from build123d import *

# Parameters (mm, degrees)
SKETCH1_R           = 3.2
BOSS_EXTRUDE1_DEPTH = 20
SKETCH3_R           = 3.2
CUT_EXTRUDE1_DEPTH  = 10
CUT_EXTRUDE2_DEPTH  = 5.5
SKETCH6_R           = 1.5
CUT_EXTRUDE4_DEPTH  = 21
CHAMFER1_SIZE       = 2
SKETCH8_R           = 1.16
CUT_EXTRUDE5_DEPTH  = 10
FILLET1_R           = 1


with BuildPart() as part:
    # Sketch1 → Boss-Extrude1 (new body)
    with BuildSketch(Plane.XY):
        with BuildLine():
            Line((20.020647688, -81), (9.925461516, 1.218693434))
            ThreePointArc((9.925461516, 1.218693434), (0, 10), (-9.925461516, 1.218693434))
            Line((-9.925461516, 1.218693434), (-20.020647688, -81))
            Line((-20.020647688, -81), (-42.020647688, -81))
            Line((-42.020647688, -81), (-42.020647688, -90))
            Line((-42.020647688, -90), (42.020647688, -90))
            Line((42.020647688, -90), (42.020647688, -81))
            Line((42.020647688, -81), (20.020647688, -81))
        make_face()
        Circle(SKETCH1_R, mode=Mode.SUBTRACT)
    extrude(amount=BOSS_EXTRUDE1_DEPTH)

    # Sketch3 → Cut-Extrude1 (cut, through all)
    with BuildSketch(Plane(origin=(0, -81, 0), x_dir=(1, 0, 0), z_dir=(0, 1, 0))):
        with Locations((-31.020647688, -10)):
            Circle(SKETCH3_R)
        with Locations((31.020647688, -10)):
            Circle(SKETCH3_R)
    extrude(amount=-CUT_EXTRUDE1_DEPTH, mode=Mode.SUBTRACT)

    # Sketch4 → Cut-Extrude2 (cut)
    with BuildSketch(Plane.XY.offset(20)):
        Polygon((0, 6.062177826), (-5.25, 3.031088913), (-5.25, -3.031088913), (0, -6.062177826), (5.25, -3.031088913), (5.25, 3.031088913), align=None)
    extrude(amount=-CUT_EXTRUDE2_DEPTH, mode=Mode.SUBTRACT)

    # Sketch6 → Cut-Extrude4 (cut, through all)
    with BuildSketch(Plane.XY.offset(20)):
        with Locations((0, -66)):
            Circle(SKETCH6_R)
        with Locations((0, -74)):
            Circle(SKETCH6_R)
        with Locations((0, -82)):
            Circle(SKETCH6_R)
    extrude(amount=-CUT_EXTRUDE4_DEPTH, mode=Mode.SUBTRACT)

    # Chamfer1
    chamfer1_edges = [part.edges().sort_by_distance(p)[0] for p in [
        (-1.5, -66, 20),
        (-1.5, -74, 20),
        (-1.5, -82, 20),
    ]]
    chamfer(chamfer1_edges, length=CHAMFER1_SIZE)

    # Sketch8 → Cut-Extrude5 (cut)
    with BuildSketch(Plane(origin=(-9.925461516, 1.218693434, 0), x_dir=(0, 0, 1), z_dir=(-0.992546152, 0.121869343, 0))):
        with Locations((10, -16.567228294)):
            Circle(SKETCH8_R)
        with Locations((10, -33.134456588)):
            Circle(SKETCH8_R)
        with Locations((10, -49.701684883)):
            Circle(SKETCH8_R)
        with Locations((10, -66.268913177)):
            Circle(SKETCH8_R)
    cut_extrude5 = extrude(amount=-CUT_EXTRUDE5_DEPTH, mode=Mode.SUBTRACT)

    # Mirror1: Cut-Extrude5 across plane
    add(cut_extrude5.mirror(Plane(origin=(0, 0, 0), x_dir=(0, 0, 1), z_dir=(1, 0, 0))), mode=Mode.SUBTRACT)

    # Fillet1
    fillet1_edges = [part.edges().sort_by_distance(p)[0] for p in [
        (-42.020647688, -81, 10),
        (-20.020647688, -81, 10),
        (20.020647688, -81, 10),
        (42.020647688, -81, 10),
    ]]
    fillet(fillet1_edges, radius=FILLET1_R)


solid = part.part
For this review, take the finished solid that the model builds, in its own axes (mm). A direction names the side the tool comes from. Coordinates: 2 decimals unless noted, no trailing zeros. Loops run counter-clockwise (first coordinate to the right, second up) from the corner with the lowest first, then second, coordinate; pieces in that order, holes last. Notation, with made-up numbers: (-23, 3.5) - (-13, 3.5) arc R12 ccw to (-13, 23.5) - close; hole circle Ø5 at (84.5, 21). An arc over 180 degrees is marked (long way). Use a Markdown table: item, result. Add a question column.
Item 1: For line 1 (Y direction, x = 0, z = 12.75); line 2 (Z direction, x = -6.5, y = -49.5); line 3 (X direction, y = -67, z = 16), list the stretches that pass through material, from the lowest coordinate up.
Item 2: We need section B-B (y = -4.5). Give the boundary of the cut face in (x, z), and give its area (3 significant figures).
Item 3: We need section D-D (z = 10). Give the number of separate pieces and of enclosed holes in the cut face, and give its area (3 significant figures).
Item 4: Tool access review of faces 1 (the face through (-5.25, 0, 17)), 2 (the face through (6.055, -49.315, 9.984)), 3 (the face through (0.806, -72.735, 9.126)): name each direction out of +Z, -Z, +X, -X, +Y, -Y from which nothing blocks a thin tool from reaching the whole face with its end or side.
Item 5: We need section A-A (x = 31.5). Give the boundary of the cut face in (y, z), and give its area (3 significant figures).
Item 6: Mouldability with a two-part tool opening along X and no side actions: class faces 4 (the face through (-9.06, -32.22, 8.84)), 5 (the face through (42.021, -86, 10)), 6 (the face through (-14.85, -38.88, 9.86)) as pulls with the +X half, pulls with the -X half, needs draft (parallel to the pull), parting line crosses it, or undercut.
Item 7: We need section C-C (y = -74). Give the boundary of the cut face in (x, z).
Item 8: Insertion check: pin 1 Ø4 at (y, z) = (-59.5, 4) entering from +X; pin 2 Ø1.6 at (y, z) = (-1, 17.5) entering from +X; pin 3 Ø12 at (x, z) = (6.5, 7) entering from +Y; pin 4 Ø1.8 at (x, y) = (0, -74) entering from +Z. Each pin has a flat end and moves straight along its axis. Give the tip position at first contact, or say it passes through.
Results list:
| question | item | result |
|---|---|---|
| 1 | line 1 | y = -90 to -83.5, -80.5 to -75.5, -72.5 to -67.5, -64.5 to -3.2, 3.2 to 10 |
| 1 | line 2 | z = 0 to 8.86, 11.14 to 20 |
| 1 | line 3 | x = -18.3 to -1.12, 1.12 to 18.3 |
| 2 | outline | (-10.63, 0) - (10.63, 0) - (10.63, 20) - (2.71, 20) - (2.71, 14.5) - (-2.71, 14.5) - (-2.71, 20) - (-10.63, 20) - close |
| 2 | area | 395 mm^2 |
| 3 | separate pieces | 3 |
| 3 | enclosed holes | 4 |
| 3 | area | 3,000 mm^2 |
| 4 | face 1 | +Z |
| 4 | face 2 | none |
| 4 | face 3 | +Z, -Z |
| 5 | outline | (-90, 0) - (-81, 0) - (-81, 6.84) - (-90, 6.84) - close; (-90, 13.16) - (-81, 13.16) - (-81, 20) - (-90, 20) - close |
| 5 | area | 123 mm^2 |
| 6 | face 4 | undercut |
| 6 | face 5 | pulls with the +X half |
| 6 | face 6 | pulls with the -X half |
| 7 | outline | (-19.16, 0) - (-1.5, 0) - (-1.5, 18) - (-3.5, 20) - (-19.16, 20) - close; (1.5, 0) - (19.16, 0) - (19.16, 20) - (3.5, 20) - (1.5, 18) - close |
| 8 | pin 1 | stops at x = 17.63 |
| 8 | pin 2 | stops at x = 10.3 |
| 8 | pin 3 | stops at y = 9.99 |
| 8 | pin 4 | passes through |
